Autodesk Fusion 360 part; units mm, degrees
sketch "Sketch1" plane through (0, 0, 0) normal (0, 1, 0) x (1, 0, 0)
  line L0 (0, 0) -> (41, 0) construction
  line L1 (41, 0) -> (41, -30) construction
  line L2 (41, -30) -> (0, -30) construction
  line L3 (0, -30) -> (0, 0) construction
  line L4 (-0.5, 0.5) -> (41.5, 0.5)
  line L5 (41.5, 0.5) -> (41.5, -30.5)
  line L6 (41.5, -30.5) -> (-0.5, -30.5)
  line L7 (-0.5, -30.5) -> (-0.5, 0.5)
  line L8 (-5, 5) -> (46, 5)
  line L9 (46, 5) -> (46, -35)
  line L10 (46, -35) -> (-5, -35)
  line L11 (-5, -35) -> (-5, 5)
  line L12 (30.5, -30.5) -> (30.5, -19.5)
  line L13 (30.5, -19.5) -> (41.5, -19.5)
  circle A0 centre (43.3031, 2.3031) radius 1.55
  circle A1 centre (-2.3031, -32.3031) radius 1.55
  circle A2 centre (-2.3031, -32.3031) radius 3.814
  circle A3 centre (43.3031, 2.3031) radius 3.814
  dimension "d1" = 41
  dimension "d2" = 30
  dimension "d3" = -0.5
  dimension "d4" = -5
  dimension "d5" = 11
  dimension "d6" = 11
  dimension "d7" = 3.1
  dimension "d8" = 3.1
  dimension "d22" = 2.55
  dimension "d23" = 2.55
  dimension "d30" = 7.6279
  dimension "d32" = 3.814
  dimension "d33" = 7.6279
extrude "Extrude1" add sketch "Sketch1" along normal blind 3.5 contours L4 L5 L6 L7 L12 L13 A2 A3 | L4 L5 A3 | L6 L7 A2
extrude "Extrude2" add sketch "Sketch1" along normal blind 14 contours L4 L7 L8 L11 A2 A3 | L4 L5 L8 L9 A3 | L6 L7 L10 L11 A2 | L5 L6 L9 L10 A2 A3
fillet "Fillet1" radius 1.5 4 edges at (46, 7, -5) (46, 7, 35) (-5, 7, -5) (-5, 7, 35)
ref_plane "WorkPlane1" through (20.5, 14, 15) normal (0, 1, 0) x (1, 0, 0)
sketch "Sketch2" plane through (0, 14, 0) normal (0, 1, 0) x (1, 0, 0)
  line L0 (41, -30) -> (0, -30)
  line L1 (41, 0) -> (41, -30)
  line L2 (41.5, 0.5) -> (41.5, -30.5)
  line L3 (41.5, -30.5) -> (-0.5, -30.5)
  line L4 (0, -30) -> (0, 0)
  line L5 (-0.5, -30.5) -> (-0.5, 0.5)
  line L6 (0, 0) -> (41, 0)
  line L7 (-0.5, 0.5) -> (41.5, 0.5)
  line L8 (-5, 5) -> (46, 5)
  line L9 (46, 5) -> (46, -35)
  line L10 (-5, -35) -> (-5, 5)
  line L11 (46, -35) -> (-5, -35)
  circle A0 centre (43.3031, 2.3031) radius 1.55
  circle A1 centre (-2.3031, -32.3031) radius 1.55
  line L12 (46, 0) -> (41.5, 0)
  line L13 (41.5, 0) -> (41.5, -19)
  line L14 (41.5, -19) -> (46, -19)
  line L15 (46, -19) -> (46, 0)
  line L16 (-0.5, 0) -> (-5, 0)
  line L17 (-5, 0) -> (-5, -19)
  line L18 (-5, -19) -> (-0.5, -19)
  line L19 (-0.5, -19) -> (-0.5, 0)
  line L20 (-5, 5) -> (13, 5)
  line L21 (13, 5) -> (13, 0)
  line L22 (13, 0) -> (-5, 0)
  line L23 (-5, 0) -> (-5, 5)
  line L24 (-0.5, -30.5) -> (-5, -30.5)
  line L25 (-5, -30.5) -> (-5, -27.5)
  line L26 (-5, -27.5) -> (-0.5, -27.5)
  line L27 (-0.5, -27.5) -> (-0.5, -30.5)
  dimension "d16" = 19
  dimension "d17" = 19
  dimension "d18" = 18
  dimension "d19" = 5
  dimension "d28" = 34.6062
  dimension "d29" = 45.6062
  dimension "d36" = 3
extrude "Extrude3" cut sketch "Sketch2" against normal blind 9.5 contours L5 L7 L8 L10 L16 L20 L21 L22 L23 | L5 L10 L16 L17 L18 L19 L22 | L5 L10 L18 L26 | L2 L9 L12 L13 L14 L15
extrude "Extrude4" cut sketch "Sketch1" along normal blind 1 contours L4 L5 L8 L9 A3 | L4 L5 A3 | L6 L7 A2 | L6 L7 L10 L11 A2 | L8 A3 | L11 A2 | L9 A3 | L10 A2
fillet "Fillet3" radius 1 4 edges at (-2.75, 4.5, 27.5) (13, 4.5, -2.75) (43.75, 4.5, 19) (43.75, 4.5, 0)
equation "d6 = d5"
equation "d9 = TOTAL_HEIGHT - WIRE_HEIGHT - 1 mm"
equation "d11 = TOTAL_HEIGHT"
equation "d22 = d7 / 2 + 1 mm"
equation "d23 = d8 / 2 + 1 mm"
equation "TOTAL_HEIGHT = 14 mm"
equation "WIRE_HEIGHT = 9.5 mm"
equation "d30 = d33"
equation "d33 = d32 * 2"
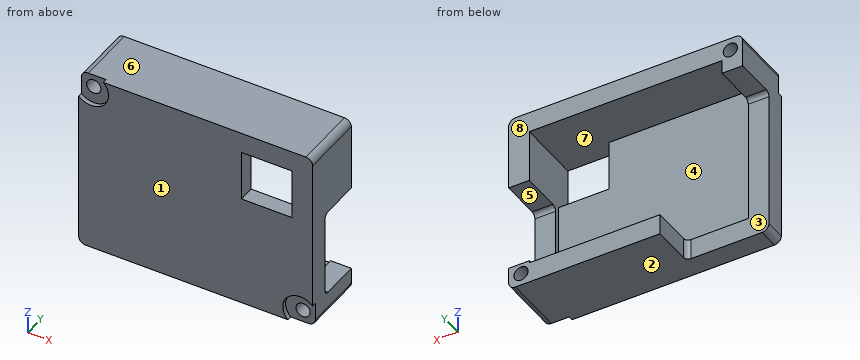
Design review of the part built by this model. Coordinates are the model's own, in mm. Face numbers are marked on the shaded views. A direction names the side the tool comes from. Give positions to 0.01 mm unless a question says otherwise; leave off trailing zeros. Write each loop counter-clockwise with the first axis right and the second up, starting at its lowest first coordinate (ties: lowest second). Pieces come first, ordered by that corner, then holes. Notation, with made-up numbers: M 24,61 L 58,61 A24 ccw 58,79 Z; hole C 35.5,-39.5 d6. An arc over 180 degrees is marked long. Return JSON: item names as keys, results as strings. Group by question number.
Item 1: The part is to be moulded in two halves that separate along Z. For the marked faces 6, 7 and 8, say which applies: pulls with the +Z half, pulls with the -Z half, needs draft (parallel to the pull), parting line crosses it, or undercut.
Item 2: Tool access review of the marked faces 1, 2, 3, 4 and 5: name each direction out of +Z, -Z, +X, -X, +Y, -Y from which nothing blocks a thin tool from reaching the whole face with its end or side.
Item 3: Take a section at A-A (x = 33). Give the boundary of the cut face in (y, z).
Item 4: Take a section at B-B (z = 25). Give the boundary of the cut face in (x, y).
Item 5: Take a section at D-D (x = 7). Give the boundary of the cut face in (y, z), plus the area to 3 significant figures.
Item 6: Wall thickness on line 1 along Z through (x, y) = (43.5, 12.5); line 2 along Z through (x, y) = (17.5, 11); line 3 along X through (y, z) = (1, 21.5): over which ranges is each line inside the solid? List them lowest first.
Item 7: Take a section at C-C (y = 12.5). Give the boundary of the cut face in (x, z).
Item 8: Clearance check with flat-ended pins moving along their axes: pin 1 Ø3.5 at (x, z) = (-2.3, 32.3) entering from -Y; pin 2 Ø13.5 at (x, z) = (2, 8.5) entering from +Y; pin 3 Ø2 at (x, z) = (-2.5, 32.5) entering from -Y; pin 4 Ø3.5 at (x, y) = (-3.5, 9.5) entering from -Z. State where each tip first meets the part, or that it passes through.
Return value:
{
 "1": {"face 6": "pulls with the +Z half", "face 7": "undercut", "face 8": "needs draft"},
 "2": {"face 1": "+Z, -Z, +X, -X, -Y", "face 2": "-Z, +X, -X, +Y, -Y", "face 3": "-Z, -X, +Y", "face 4": "+Y", "face 5": "+X, -X, +Y"},
 "3": {"outline": "M 0,-5 L 14,-5 L 14,-0.5 L 3.5,-0.5 L 3.5,19.5 L 0,19.5 Z; M 0,30.5 L 14,30.5 L 14,35 L 0,35 Z"},
 "4": {"outline": "M -5,0 L 30.5,0 L 30.5,3.5 L -0.5,3.5 L -0.5,4.5 L -5,4.5 Z; M 41.5,0 L 46,0 L 46,14 L 41.5,14 Z"},
 "5": {"outline": "M 0,-5 L 4.5,-5 L 4.5,-0.5 L 3.5,-0.5 L 3.5,30.5 L 14,30.5 L 14,35 L 0,35 Z", "area": "192 mm2"},
 "6": {"line 1": "z = -5 to -3.84, -0.77 to 0, 19 to 35", "line 2": "z = -5 to -0.5, 30.5 to 35", "line 3": "x = -5 to 30.5, 41.5 to 46"},
 "7": {"outline": "M -5,27.5 L -0.5,27.5 L -0.5,30.5 L 41.5,30.5 L 41.5,19 L 46,19 L 46,33.5 A1.5 ccw 44.5,35 L -3.5,35 A1.5 ccw -5,33.5 Z; M 13,-5 L 44.5,-5 A1.5 ccw 46,-3.5 L 46,0 L 41.5,0 L 41.5,-0.5 L 13,-0.5 Z; hole C -2.3,32.3 d3.1; hole C 43.3,-2.3 d3.1"},
 "8": {"pin 1": "stops at y = 1", "pin 2": "stops at y = 4.5", "pin 3": "passes through", "pin 4": "stops at z = 27.5"}
}
